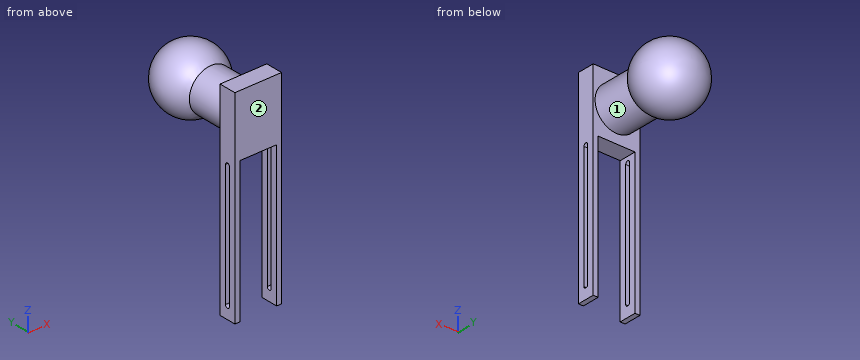
```python
from build123d import *

# Parameters (mm, degrees)
BOSS_EXTRUDE1_DEPTH = 17.78
SKETCH3_R           = 22.225
BOSS_EXTRUDE2_DEPTH = 63.5
CUT_EXTRUDE1_DEPTH  = 185.154379258


with BuildPart() as part:
    # Sketch1 → Boss-Extrude1 (new body)
    with BuildSketch(Plane(origin=(0, 0, 0), x_dir=(1, 0, 0), z_dir=(0, 1, 0))):
        Polygon((-19.05, 146.05), (-24.13, 146.05), (-24.13, -63.5), (24.13, -63.5), (24.13, 146.05), (19.05, 146.05), (19.05, 0), (-19.05, 0), align=None)
    extrude(amount=-BOSS_EXTRUDE1_DEPTH)

    # Sketch3 → Boss-Extrude2 (add)
    with BuildSketch(Plane(origin=(0, 0, 0), x_dir=(1, 0, 0), z_dir=(0, 1, 0))):
        with Locations(Location((0, -31.75, 0), (0, 0, 270))):
            Circle(SKETCH3_R)
    extrude(amount=BOSS_EXTRUDE2_DEPTH)

    # Sketch5 → Revolve1 (revolve)
    with BuildSketch(Plane(origin=(0, 0, 31.75), x_dir=(0, -1, 0), z_dir=(0, 0, 1))):
        with BuildLine():
            Line((-63.5, -33.02), (-63.5, 33.02))
            ThreePointArc((-63.5, 33.02), (-96.52, 0), (-63.5, -33.02))
        make_face()
    revolve(axis=Axis((0, 63.5, 31.75), (1, 0, 0)))

    # Sketch6 → Cut-Extrude1 (cut, through all)
    with BuildSketch(Plane.ZY.offset(24.13)):
        with BuildLine():
            Line((-133.35, -6.604), (-6.35, -6.604))
            ThreePointArc((-6.35, -6.604), (-4.064, -8.89), (-6.35, -11.176))
            Line((-6.35, -11.176), (-133.35, -11.176))
            ThreePointArc((-133.35, -11.176), (-135.636, -8.89), (-133.35, -6.604))
        make_face()
    extrude(amount=-CUT_EXTRUDE1_DEPTH, mode=Mode.SUBTRACT)


solid = part.part
```
Part model, mm, in its own coordinate system. Face numbers are marked on the shaded views. A direction names the side the tool comes from. Coordinates: 2 decimals unless noted, no trailing zeros. Loops run counter-clockwise (first coordinate to the right, second up) from the corner with the lowest first, then second, coordinate; pieces in that order, holes last. Notation, with made-up numbers: (32.25, 5) - (51.25, 5) arc R26 ccw to (51.25, 32) - close; hole circle Ø11 at (35, 34). An arc over 180 degrees is marked (long way). Write item = value, one per line. Start each with the question number.
Item 1: Cut at B-B, the plane z = -18. Give the cut face in (x, y).
Item 2: Cut at D-D, the plane x = 0. Give the cut face in (y, z) (3 decimals), and give its area (3 significant figures).
Item 3: Wall check: L1, parallel to Z at x = 1, y = 30; L2, parallel to Y at x = 10, z = 53; L3, parallel to Y at x = 26, z = 34.5. Give the ranges that are in metal, low to high. Write a range as from..to.
Item 4: Cut at A-A, the plane y = -8.89. Give the cut face in (x, z), and give its area (3 significant figures).
Item 5: Flat gauge pins, fed straight in: pin 1 Ø5.5 at (y, z) = (-5.5, -89.5) entering from -X; pin 2 Ø4 at (x, y) = (-23.5, 1.5) entering from -Z; pin 3 Ø6 at (x, y) = (-7.5, 53) entering from +Z; pin 4 Ø12 at (x, z) = (-24, 23) entering from +Y. Where does each tip first touch, or does it go through?
Item 6: Cut at C-C, the plane z = 31.75. Give the cut face in (x, y) (3 decimals).
Item 7: 3-axis set-ups, long thin cutter, end or side, ignore diameter. For the marked faces 1 and 2: which of +Z, -Z, +X, -X, +Y, -Y reach the whole face in a straight line?
The answers:
q1.outline = (-24.13, -17.78) - (-19.05, -17.78) - (-19.05, -11.18) - (-24.13, -11.18) - close; (-24.13, -6.6) - (-19.05, -6.6) - (-19.05, 0) - (-24.13, 0) - close; (19.05, -17.78) - (24.13, -17.78) - (24.13, -11.18) - (19.05, -11.18) - close; (19.05, -6.6) - (24.13, -6.6) - (24.13, 0) - (19.05, 0) - close
q2.outline = (-17.78, 0) - (0, 0) - (0, 9.525) - (39.079, 9.525) arc R33.02 ccw (long way) to (39.079, 53.975) - (0, 53.975) - (0, 63.5) - (-17.78, 63.5) - close
q2.area = 6,030 mm2
q3.L1 = 9.55..53.95
q3.L2 = -17.78..0, 40.29..86.71
q3.L3 = 43.33..83.67
q4.outline = (-24.13, -146.05) - (-19.05, -146.05) - (-19.05, -135.64) - (-24.13, -135.64) - close; (-24.13, -4.06) - (-19.05, -4.06) - (-19.05, 0) - (19.05, 0) - (19.05, -4.06) - (24.13, -4.06) - (24.13, 63.5) - (-24.13, 63.5) - close; (19.05, -146.05) - (24.13, -146.05) - (24.13, -135.64) - (19.05, -135.64) - close
q4.area = 3,210 mm2
q5.pin_1 = -24.13
q5.pin_2 = -146.05
q5.pin_3 = 63.25
q5.pin_4 = 90.11
q6.outline = (-24.13, -17.78) - (24.13, -17.78) - (24.13, 0) - (22.225, 0) - (22.225, 39.079) arc R33.02 ccw (long way) to (-22.225, 39.079) - (-22.225, 0) - (-24.13, 0) - close
q7.face_1 = none
q7.face_2 = +Z, -Z, +X, -X, -Y
